from build123d import *

# Parameters (mm, degrees)
F0_W     = 203.2
F0_H     = 101.6
F1_DEPTH = 12.7
F2_D     = 14.2875
F4_W     = 203.2
F4_H     = 101.6
F5_DEPTH = 12.7
F6_W     = 101.6
F6_H     = 269.748
F7_DEPTH = 6.35


with BuildPart() as f1:
    # F0 (on Top) → F1 (new body)
    with BuildSketch(Plane.XY):
        Rectangle(F0_W, F0_H)
    extrude(amount=F1_DEPTH)

    # F2 (through all)
    with Locations(Plane(origin=(0, 0, 0), x_dir=(1, 0, 0), z_dir=(0, 0, -1))):
        with Locations((-76.2, 25.4), (-76.2, -25.4), (76.2, -25.4), (76.2, 25.4)):
            Hole(F2_D / 2)



with BuildPart() as f5:
    # F4 (on offset) → F5 (new body)
    with BuildSketch(Plane.XY.offset(295.148)):
        Rectangle(F4_W, F4_H)
        with BuildLine():
            Line((-65.913, -38.1), (-65.913, 38.1))
            ThreePointArc((-65.913, 38.1), (-60.325, 43.688), (-54.737, 38.1))
            Line((-54.737, 38.1), (-54.737, -38.1))
            ThreePointArc((-54.737, -38.1), (-60.325, -43.688), (-65.913, -38.1))
        make_face(mode=Mode.SUBTRACT)
        with BuildLine():
            ThreePointArc((54.737, 38.1), (60.325, 43.688), (65.913, 38.1))
            Line((65.913, 38.1), (65.913, -38.1))
            ThreePointArc((65.913, -38.1), (60.325, -43.688), (54.737, -38.1))
            Line((54.737, -38.1), (54.737, 38.1))
        make_face(mode=Mode.SUBTRACT)
    extrude(amount=-F5_DEPTH)


with BuildPart() as f1_1:
    add(f1.part)

    add(f5.part)  # F7 merges F5
    # F6 (on face) → F7 (join, symmetric)
    with BuildSketch(Plane.YZ.offset(101.6)):
        with Locations((0, 147.574)):
            Rectangle(F6_W, F6_H)
    extrude(amount=F7_DEPTH, both=True)

    # F8: F1 across plane


with BuildPart() as f1_2:
    add(f1_1.part)
    add(f1_1.part.mirror(Plane.YZ))


solid = f1_2.part
Geometry check sheet. Reference: the model listing, model coordinates, mm. A direction names the side the tool comes from. Round coordinates to 2 decimals unless told otherwise and drop trailing zeros. Loops run counter-clockwise (first coordinate to the right, second up) from the corner with the lowest first, then second, coordinate; pieces in that order, holes last. Notation, with made-up numbers: (9.25, 88.25) -> (25.25, 88.25) arc R32 ccw to (25.25, 118.25) -> close; hole circle Ø7 at (66, 34). An arc over 180 degrees is marked (long way). Answer as a JSON object with one key per item and string values. Group by question number.
Item 1: Thickness scan on line 1 along X through (y, z) = (-25.4, 4.75); line 2 along Y through (x, z) = (76, 6); line 3 along Z through (x, y) = (-1, 33.5). Record the ranges inside material, lowest first.
Item 2: Cross-section at B-B, the plane x = 28.5. Record the cut outline in (y, z).
Item 3: Set-up check for faces 4 (the face through (101.6, -1, 289)), 5 (the face through (95.25, -1, 149)), 6 (the face through (65.913, 1, 289)), 7 (the face through (-83.014, -27.546, 6.439)): record each of +Z, -Z, +X, -X, +Y, -Y from which the full face is reachable in a straight line by a thin tool's end or side.
Item 4: Depth check by flat-ended pin: pin 1 Ø4 at (y, z) = (0.5, 287.5) entering from +X; pin 2 Ø5 at (x, y) = (-104.5, 4) entering from -Z; pin 3 Ø3 at (x, y) = (-103.5, 2.5) entering from +Z. Enter the tip coordinate at first touch or a pass-through.
Item 5: Release check for a two-part mould opening along Y. For faces 1 (the face through (-95.25, -1, 149)), 2 (the face through (-95.5, 50.8, 136)), 3 (the face through (-60.202, -43.687, 288.887)) record: pulls with the +Y half, pulls with the -Y half, needs draft (parallel to the pull), parting line crosses it, or undercut.
Item 6: Cross-section at C-C, the plane z = 177.5. Record the cut outline in (x, y).
Item 7: Cross-section at A-A, the plane y = 2. Record the cut outline in (x, z), plus the area to 3 significant figures.
Item 8: Cross-section at D-D, the plane y = -25.4. Count the separate pieces of the cut face and the enclosed holes in it, plus the area to 3 significant figures.
Determined:
{
 "1": {"line 1": "x = -101.6 to -83.34, -69.06 to 69.06, 83.34 to 101.6", "line 2": "y = -50.8 to -32.54, -18.26 to 18.26, 32.54 to 50.8", "line 3": "z = 0 to 12.7, 282.45 to 295.15"},
 "2": {"outline": "(-50.8, 0) -> (50.8, 0) -> (50.8, 12.7) -> (-50.8, 12.7) -> close; (-50.8, 282.45) -> (50.8, 282.45) -> (50.8, 295.15) -> (-50.8, 295.15) -> close"},
 "3": {"face 4": "+Z, +X, +Y, -Y", "face 5": "+Y, -Y", "face 6": "+Z", "face 7": "-Z"},
 "4": {"pin 1": "stops at x = 101.6", "pin 2": "stops at z = 12.7", "pin 3": "stops at z = 282.45"},
 "5": {"face 1": "needs draft", "face 2": "pulls with the +Y half", "face 3": "undercut"},
 "6": {"outline": "(-107.95, -50.8) -> (-95.25, -50.8) -> (-95.25, 50.8) -> (-107.95, 50.8) -> close; (95.25, -50.8) -> (107.95, -50.8) -> (107.95, 50.8) -> (95.25, 50.8) -> close"},
 "7": {"outline": "(-107.95, 12.7) -> (-101.6, 12.7) -> (-101.6, 0) -> (101.6, 0) -> (101.6, 12.7) -> (107.95, 12.7) -> (107.95, 282.45) -> (101.6, 282.45) -> (101.6, 295.15) -> (65.91, 295.15) -> (65.91, 282.45) -> (95.25, 282.45) -> (95.25, 12.7) -> (-95.25, 12.7) -> (-95.25, 282.45) -> (-65.91, 282.45) -> (-65.91, 295.15) -> (-101.6, 295.15) -> (-101.6, 282.45) -> (-107.95, 282.45) -> close; (-54.74, 282.45) -> (54.74, 282.45) -> (54.74, 295.15) -> (-54.74, 295.15) -> close", "area": "11,700 mm²"},
 "8": {"separate pieces": "4", "enclosed holes": "0", "area": "11,400 mm²"}
}
